For this review, take the finished solid that the model builds, in its own axes (mm). Give positions to 0.01 mm unless a question says otherwise; leave off trailing zeros. Loops run counter-clockwise (first coordinate to the right, second up) from the corner with the lowest first, then second, coordinate; pieces in that order, holes last. Notation, with made-up numbers: (-40, 62.25) - (-5, 62.25) arc R16 ccw to (-5, 82.25) - close; hole circle Ø7 at (-18, -24). An arc over 180 degrees is marked (long way). Use CSV: the item, a comma, the result in double quotes. Start each with the question number.
1. Take a section at A-A on x = 8.5. Give the boundary of the cut face in (y, z).
2. Take a section at C-C on z = 3.1. Give the boundary of the cut face in (x, y).
3. Take a section at B-B on y = 37.5. Give the boundary of the cut face in (x, z).
4. Wall thickness on line 1 (Y direction, x = 12, z = 1.3); line 2 (X direction, y = 114.5, z = 1.35); line 3 (Y direction, x = 165, z = 3.35): over which ranges is each line inside the solid? List them lowest first.
5. For pin 1 (1.5 mm diameter, centred on y = -34.5, z = 2.5, fed in from +X); pin 2 (1.5 mm diameter, centred on x = 37, z = 2.5, fed in from -Y), all flat-tipped, find the tip position at first contact; note any pin that passes through.
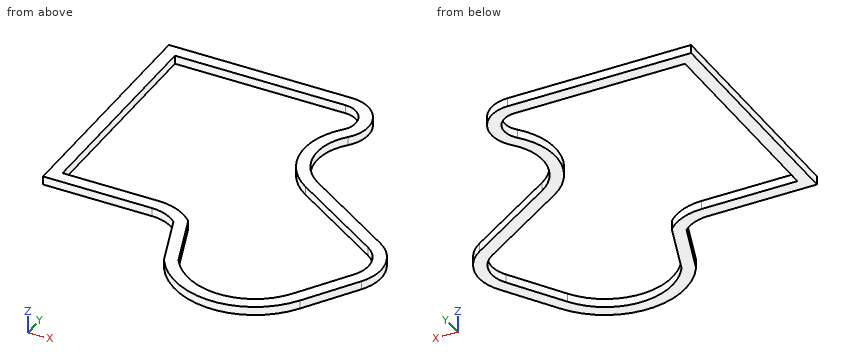
```python
from build123d import *

# Parameters (mm, degrees)
BOSS_EXTRUDE1_DEPTH = 5.08


with BuildPart() as part:
    # Sketch1 → Boss-Extrude1 (new body)
    with BuildSketch(Plane.XY):
        with BuildLine():
            Line((-7.62, -7.62), (-7.62, 134.62))
            Line((-7.62, 134.62), (101.6, 134.62))
            ThreePointArc((101.6, 134.62), (120.252989831, 122.555420822), (116.89921922, 100.595449896))
            ThreePointArc((116.89921922, 100.595449896), (109.507548694, 76.190999841), (123.247106812, 54.709879795))
            Line((123.247106812, 54.709879795), (179.49628154, 18.640745596))
            ThreePointArc((179.49628154, 18.640745596), (191.154782754, 1.885366153), (187.550745596, -18.20628154))
            Line((187.550745596, -18.20628154), (167.450498742, -49.552259826))
            ThreePointArc((167.450498742, -49.552259826), (126.559009674, -71.664336239), (86.0802479, -48.805472603))
            Line((86.0802479, -48.805472603), (73.370195116, -13.884889578))
            ThreePointArc((73.370195116, -13.884889578), (65.844014766, -9.240646228), (57.15, -7.62))
            Line((57.15, -7.62), (-7.62, -7.62))
        make_face()
        with BuildLine():
            Line((0, 0), (0, 127))
            Line((0, 127), (101.6, 127))
            ThreePointArc((101.6, 127), (113.303244129, 119.430451273), (111.199024024, 105.65234368))
            ThreePointArc((111.199024024, 105.65234368), (101.959435867, 75.14678111), (119.133883514, 48.295381054))
            Line((119.133883514, 48.295381054), (175.383058243, 12.226246854))
            ThreePointArc((175.383058243, 12.226246854), (183.71055911, 0.258118681), (181.136246854, -14.093058243))
            Line((181.136246854, -14.093058243), (161.036, -45.439036529))
            ThreePointArc((161.036, -45.439036529), (127, -64.046359823), (92.964, -45.439036529))
            Line((92.964, -45.439036529), (79.933032539, -9.636747677))
            ThreePointArc((79.933032539, -9.636747677), (69.518644605, -2.508263892), (57.15, 0))
            Line((57.15, 0), (0, 0))
        make_face(mode=Mode.SUBTRACT)
    extrude(amount=BOSS_EXTRUDE1_DEPTH)


solid = part.part
```
Check result:
1,outline,"(-7.62, 0) - (0, 0) - (0, 5.08) - (-7.62, 5.08) - close; (127, 0) - (134.62, 0) - (134.62, 5.08) - (127, 5.08) - close"
2,outline,"(-7.62, -7.62) - (57.15, -7.62) arc R24.13 cw to (73.37, -13.88) - (86.08, -48.81) arc R48.05 ccw to (167.45, -49.55) - (187.55, -18.21) arc R26.67 ccw to (179.5, 18.64) - (123.25, 54.71) arc R30.48 cw to (116.9, 100.6) arc R20.45 ccw to (101.6, 134.62) - (-7.62, 134.62) - close; hole (0, 0) - (57.15, 0) arc R31.75 cw to (79.93, -9.64) - (92.96, -45.44) arc R40.43 ccw to (161.04, -45.44) - (181.14, -14.09) arc R19.05 ccw to (175.38, 12.23) - (119.13, 48.3) arc R38.1 cw to (111.2, 105.65) arc R12.83 ccw to (101.6, 127) - (0, 127) - close"
3,outline,"(-7.62, 0) - (0, 0) - (0, 5.08) - (-7.62, 5.08) - close; (135.97, 0) - (150.09, 0) - (150.09, 5.08) - (135.97, 5.08) - close"
4,line 1,"y = -7.62 to 0, 127 to 134.62"
4,line 2,"x = -7.62 to 0, 114.43 to 122.05"
4,line 3,"y = -53.03 to -39.26, 18.88 to 27.94"
5,pin 1,"stops at x = 177.58"
5,pin 2,"stops at y = -7.62"
